from build123d import *

# Parameters (mm, degrees)
SKETCH2_W            = 18.7
SKETCH2_H            = 20
BOSS_EXTRUDE1_DEPTH  = 25.4
SKETCH3_W            = 6.35
SKETCH3_H            = 3.175
SKETCH3_H_2          = 4.125
CUT_EXTRUDE1_DEPTH   = 34.653863077
SKETCH5_W            = 3.175
SKETCH5_H            = 25.4
BOSS_EXTRUDE2_DEPTH  = 20
SKETCH6_W            = 10
SKETCH6_H            = 10.125
CUT_EXTRUDE2_DEPTH   = 16.825
CUT_EXTRUDE3_REACH   = 34.439
SKETCH7_W            = 3
SKETCH7_H            = 3.5
SKETCH8_W            = 22
SKETCH8_H            = 10.125
CUT_EXTRUDE4_DEPTH   = 19
BOSS_EXTRUDE3_REACH  = 39.049
SKETCH10_W           = 3.175
SKETCH10_H           = 20.1625
BOSS_EXTRUDE10_REACH = 39.695
CUT_EXTRUDE5_REACH   = 33.235
SKETCH12_W           = 6.175
SKETCH12_H           = 10.825
BOSS_EXTRUDE11_REACH = 33.235


with BuildPart() as part:
    # Sketch2 → Boss-Extrude1 (new body)
    with BuildSketch(Plane(origin=(0, 0, 0), x_dir=(1, 0, 0), z_dir=(0, 1, 0))):
        Rectangle(SKETCH2_W, SKETCH2_H)
    extrude(amount=BOSS_EXTRUDE1_DEPTH)

    # Sketch3 → Cut-Extrude1 (cut, through all)
    with BuildSketch(Plane(origin=(0, 0, -10), x_dir=(-1, 0, 0), z_dir=(0, 0, -1))):
        with Locations((0, 16.5125)):
            Rectangle(SKETCH3_W, SKETCH3_H)
        with Locations((0, 20.1625)):
            Rectangle(SKETCH3_W, SKETCH3_H_2)
        with Locations((0, 23.8125)):
            Rectangle(SKETCH3_W, SKETCH3_H)
    extrude(amount=-CUT_EXTRUDE1_DEPTH, mode=Mode.SUBTRACT)

    # Sketch5 → Boss-Extrude2 (add)
    with BuildSketch(Plane(origin=(0, 0, -10), x_dir=(-1, 0, 0), z_dir=(0, 0, -1))):
        with Locations((-10.9375, 12.7)):
            Rectangle(SKETCH5_W, SKETCH5_H)
        with Locations((10.9375, 12.7)):
            Rectangle(SKETCH5_W, SKETCH5_H)
    extrude(amount=-BOSS_EXTRUDE2_DEPTH)

    # Sketch6 → Cut-Extrude2 (cut)
    with BuildSketch(Plane(origin=(0, 0, -10), x_dir=(-1, 0, 0), z_dir=(0, 0, -1))):
        Polygon((5, 22.225), (5, 10.125), (5, 0), (9.35, 0), (9.35, 22.225), align=None)
        with Locations((0, 5.0625)):
            Rectangle(SKETCH6_W, SKETCH6_H)
        Polygon((-5, 22.225), (-9.35, 22.225), (-9.35, 0), (-5, 0), (-5, 10.125), align=None)
    extrude(amount=-CUT_EXTRUDE2_DEPTH, mode=Mode.SUBTRACT)

    # Cut-Extrude3: up to this face of the body (flat: up to its plane)
    cut_extrude3_end = Plane(part.part.faces().sort_by_distance((-5, 16.175, -1.5875))[0])
    # Sketch7 → Cut-Extrude3 (cut, up to the picked face)
    with BuildSketch(Plane(origin=(5, 0, 0), x_dir=(0, 0, -1), z_dir=(1, 0, 0)), mode=Mode.PRIVATE) as cut_extrude3_sk1:
        with Locations((-4.825, 19.225)):
            Rectangle(SKETCH7_W, SKETCH7_H)
    cut_extrude3_tool1 = split(extrude(cut_extrude3_sk1.sketch, amount=-CUT_EXTRUDE3_REACH, mode=Mode.PRIVATE), bisect_by=cut_extrude3_end, keep=Keep.BOTH, mode=Mode.PRIVATE)
    add(cut_extrude3_tool1.solids().sort_by(Axis((5, 19.225, 4.825), (-1, 0, 0)))[0], mode=Mode.SUBTRACT)

    # Sketch8 → Cut-Extrude4 (cut)
    with BuildSketch(Plane(origin=(0, 0, -10), x_dir=(-1, 0, 0), z_dir=(0, 0, -1))):
        with Locations((0, 5.0625)):
            Rectangle(SKETCH8_W, SKETCH8_H)
    extrude(amount=-CUT_EXTRUDE4_DEPTH, mode=Mode.SUBTRACT)

    # Boss-Extrude3: up to this face of the body (flat: up to its plane)
    boss_extrude3_end = Plane(part.part.faces().sort_by_distance((-12.525, 12.7, 0))[0])
    # Sketch10 → Boss-Extrude3 (add, up to the picked face)
    with BuildSketch(Plane(origin=(12.525, 0, 0), x_dir=(0, 0, -1), z_dir=(1, 0, 0)), mode=Mode.PRIVATE) as boss_extrude3_sk1:
        with Locations((-10.5875, 10.08125)):
            Rectangle(SKETCH10_W, SKETCH10_H)
    boss_extrude3_tool1 = split(extrude(boss_extrude3_sk1.sketch, amount=-BOSS_EXTRUDE3_REACH, mode=Mode.PRIVATE), bisect_by=boss_extrude3_end, keep=Keep.BOTH, mode=Mode.PRIVATE)
    add(boss_extrude3_tool1.solids().sort_by(Axis((12.525, 10.08125, 10.5875), (-1, 0, 0)))[0])

    # Boss-Extrude10: up to this face of the body (flat: up to its plane)
    boss_extrude10_end = Plane(part.part.faces().sort_by_distance((-12.525, 12.491899114, 0.881076306))[0])
    # Sketch11 → Boss-Extrude10 (add, up to the picked face)
    with BuildSketch(Plane(origin=(12.525, 0, 0), x_dir=(0, 0, -1), z_dir=(1, 0, 0)), mode=Mode.PRIVATE) as boss_extrude10_sk1:
        Polygon((-0.825, 16.939816253), (-0.825, 12.910183747), (10, 21.370367494), (10, 25.4), align=None)
    boss_extrude10_tool1 = split(extrude(boss_extrude10_sk1.sketch, amount=-BOSS_EXTRUDE10_REACH, mode=Mode.PRIVATE), bisect_by=boss_extrude10_end, keep=Keep.BOTH, mode=Mode.PRIVATE)
    # Sketch11 → Boss-Extrude10 (add, up to the picked face)
    with BuildSketch(Plane(origin=(12.525, 0, 0), x_dir=(0, 0, -1), z_dir=(1, 0, 0)), mode=Mode.PRIVATE) as boss_extrude10_sk2:
        Polygon((13.175, 0), (10, 0), (10, 25.4), (10, 44.45), (13.175, 44.45), align=None)
    boss_extrude10_tool2 = split(extrude(boss_extrude10_sk2.sketch, amount=-BOSS_EXTRUDE10_REACH, mode=Mode.PRIVATE), bisect_by=boss_extrude10_end, keep=Keep.BOTH, mode=Mode.PRIVATE)
    add(boss_extrude10_tool1.solids().sort_by(Axis((12.525, 19.155092, -4.5875), (-1, 0, 0)))[0])
    add(boss_extrude10_tool2.solids().sort_by(Axis((12.525, 22.225, -11.5875), (-1, 0, 0)))[0])

    # Cut-Extrude5: up to this face of the body (flat: up to its plane)
    cut_extrude5_end = Plane(part.part.faces().sort_by_distance((0, 21.169908126, -4.5875))[0])
    # Sketch12 → Cut-Extrude5 (cut, up to the picked face)
    with BuildSketch(Plane(origin=(0, 25.4, 0), x_dir=(1, 0, 0), z_dir=(0, 1, 0)), mode=Mode.PRIVATE) as cut_extrude5_sk1:
        Polygon((-3.175, 10), (-9.35, 10), (-9.35, 3.175), (-3.175, -0.825), align=None)
    cut_extrude5_tool1 = split(extrude(cut_extrude5_sk1.sketch, amount=-CUT_EXTRUDE5_REACH, mode=Mode.PRIVATE), bisect_by=cut_extrude5_end, keep=Keep.BOTH, mode=Mode.PRIVATE)
    # Sketch12 → Cut-Extrude5 (cut, up to the picked face)
    with BuildSketch(Plane(origin=(0, 25.4, 0), x_dir=(1, 0, 0), z_dir=(0, 1, 0)), mode=Mode.PRIVATE) as cut_extrude5_sk2:
        with Locations((6.2625, 4.5875)):
            Rectangle(SKETCH12_W, SKETCH12_H)
    cut_extrude5_tool2 = split(extrude(cut_extrude5_sk2.sketch, amount=-CUT_EXTRUDE5_REACH, mode=Mode.PRIVATE), bisect_by=cut_extrude5_end, keep=Keep.BOTH, mode=Mode.PRIVATE)
    add(cut_extrude5_tool1.solids().sort_by(Axis((-6.029261, 25.4, -5.511957), (0, -1, 0)))[0], mode=Mode.SUBTRACT)
    add(cut_extrude5_tool2.solids().sort_by(Axis((6.2625, 25.4, -4.5875), (0, -1, 0)))[0], mode=Mode.SUBTRACT)

    # Boss-Extrude11: up to this plane
    boss_extrude11_end = Plane(origin=(-59.127601859, 10.916634462, 8.531799857), z_dir=(0, 0.7879130405339252, 0.6157865219023434))
    # Sketch13 → Boss-Extrude11 (add, up to the surface)
    with BuildSketch(Plane(origin=(0, 25.4, 0), x_dir=(1, 0, 0), z_dir=(0, 1, 0)), mode=Mode.PRIVATE) as boss_extrude11_sk1:
        Polygon((-9.35, 3.175), (-9.35, -0.825), (-3.175, -0.825), align=None)
    boss_extrude11_tool1 = split(extrude(boss_extrude11_sk1.sketch, amount=-BOSS_EXTRUDE11_REACH, mode=Mode.PRIVATE), bisect_by=boss_extrude11_end, keep=Keep.BOTH, mode=Mode.PRIVATE)
    add(boss_extrude11_tool1.solids().sort_by_distance((-7.291667, 25.4, -0.508333))[0])
    # Sketch13 → Boss-Extrude11 (add, up to the surface)
    with BuildSketch(Plane(origin=(0, 25.4, 0), x_dir=(1, 0, 0), z_dir=(0, 1, 0)), mode=Mode.PRIVATE) as boss_extrude11_sk2:
        Polygon((9.35, 3.175), (9.35, -0.825), (3.175, -0.825), align=None)
    boss_extrude11_tool2 = split(extrude(boss_extrude11_sk2.sketch, amount=-BOSS_EXTRUDE11_REACH, mode=Mode.PRIVATE), bisect_by=boss_extrude11_end, keep=Keep.BOTH, mode=Mode.PRIVATE)
    add(boss_extrude11_tool2.solids().sort_by_distance((7.291667, 25.4, -0.508333))[0])


solid = part.part
Geometry check sheet. Reference: the model listing, model coordinates, mm. A direction names the side the tool comes from. Round coordinates to 2 decimals unless told otherwise and drop trailing zeros. Loops run counter-clockwise (first coordinate to the right, second up) from the corner with the lowest first, then second, coordinate; pieces in that order, holes last. Notation, with made-up numbers: (43.5, -10.5) - (90.5, -10.5) arc R29 ccw to (90.5, 12.5) - close; hole circle Ø3 at (-15.75, 40.25). An arc over 180 degrees is marked (long way). One line per question, with ' | ' between items. Start each with the question number.
1. Scan lines: line 1 (X direction, y = 12.5, z = 0.25) (3 decimals); line 2 (X direction, y = 15, z = 6.75) (3 decimals); line 3 (Z direction, x = -7.25, y = 10) (3 decimals). Record each from-to range of solid material in increasing order. Write a range as [from, to].
2. Cross-section at B-B on y = 7.5. Record the cut outline in (x, z) (3 decimals), then the cut area to 3 significant figures.
3. Cross-section at A-A on z = 5.5. Record the cut outline in (x, y) (3 decimals), then the cut area to 3 significant figures.
4. Depth check by flat-ended pin: pin 1 (4.5 mm diameter, centred on x = 6.5, z = 1, fed in from +Y); pin 2 (3.5 mm diameter, centred on x = 7, z = 3, fed in from -Y) (3 decimals); pin 3 (3 mm diameter, centred on x = 0, z = 3, fed in from +Y) (3 decimals). Enter the tip coordinate at first touch or a pass-through.
5. Draft check along Z on faces 1 (the face through (8, 23, 10)), 2 (the face through (0, 10.125, -1)), 3 (the face through (9, 25.4, 2)). Enter one of: released by +Z, released by -Z, zero draft, split by the parting line, or undercut.
6. Tool access check on faces 4 (the face through (4, 20.975, 5)), 5 (the face through (0.13, 22.17, -5.87)), 6 (the face through (-11, 5, -1)). Record the directions out of +Z, -Z, +X, -X, +Y, -Y that give a thin tool (end or side, any length) a straight path to the whole face; none if there is none.
Taken from the geometry:
1) line 1: [-12.525, -9.35], [-5, 5], [9.35, 12.525] | line 2: [-12.525, -9.35], [-5, -3.175], [3.175, 5], [9.35, 12.525] | line 3: [-13.175, -10], [9, 12.175]
2) outline: (-12.525, -13.175) - (12.525, -13.175) - (12.525, 12.175) - (-12.525, 12.175) - close; hole (-11, -10) - (11, -10) - (11, 9) - (-11, 9) - close | area: 217 mm²
3) outline: (-12.525, 0) - (-11, 0) - (-11, 10.125) - (-9.35, 10.125) - (-9.35, 22.225) - (-5, 22.225) - (-5, 20.975) - (-3.175, 20.975) - (-3.175, 25.4) - (-12.525, 25.4) - close; (-5, 10.125) - (5, 10.125) - (5, 17.475) - (3.175, 17.475) - (3.175, 14.925) - (-3.175, 14.925) - (-3.175, 17.475) - (-5, 17.475) - close; (3.175, 20.975) - (5, 20.975) - (5, 22.225) - (9.35, 22.225) - (9.35, 10.125) - (11, 10.125) - (11, 0) - (12.525, 0) - (12.525, 25.4) - (3.175, 25.4) - close | area: 229 mm²
4) pin 1: y = 25.4 | pin 2: y = 22.225 | pin 3: y = 14.925
5) face 1: released by +Z | face 2: undercut | face 3: zero draft
6) face 4: none | face 5: +Y | face 6: -Y
